For this review, take the finished solid that the model builds, in its own axes (mm). A direction names the side the tool comes from. Coordinates: 2 decimals unless noted, no trailing zeros. Loops run counter-clockwise (first coordinate to the right, second up) from the corner with the lowest first, then second, coordinate; pieces in that order, holes last. Notation, with made-up numbers: M 72.25,45.5 L 118.25,45.5 A17 ccw 118.25,68.5 Z; hole C -8,75 d9. An arc over 180 degrees is marked long. Answer as a JSON object with one key per item and string values. Group by question number.
Item 1: Add section B-B (y = 0). State the section outline as (x, z) points.
Item 2: Add section A-A (z = 6). State the section outline as (x, y) points.
Item 3: Tool access review of faces 1 (the face through (-13, -13, 20.7)), 2 (the face through (-17.8, 17.87, 10.49)): name each direction out of +Z, -Z, +X, -X, +Y, -Y from which nothing blocks a thin tool from reaching the whole face with its end or side.
Item 4: Mouldability with a two-part tool opening along Y and no side actions: class faces 3 (the face through (19.3, 0, 10)), 4 (the face through (17.264, -5.437, 26.468)), 5 (the face through (15.209, -13.523, 10.495)), 6 (the face through (-12.991, -13.523, 10.495)) as +Y half, -Y half, draft (parallel to the pull), parting line (faces both ways), or undercut.
Item 5: Wall thickness on L1, parallel to Y at x = 14.1, z = 5.5; L2, parallel to X at y = 15, z = 12.5: over which ranges is each line inside the solid? List them lowest first. Write a range as from..to.
Item 6: Insertion check: pin 1 (4 mm diameter, centred on x = -14.1, y = -14.1, fed in from +Z); pin 2 (2 mm diameter, centred on x = 14.1, y = -14.1, fed in from +Z); pin 3 (6 mm diameter, centred on x = 11, z = 30, fed in from +Y). Each pin has a flat end and moves straight along its axis. Give the tip position at first contact, or say it passes through.
Autodesk Inventor part; units mm, degrees
ref_plane "YZ Plane" through (0, 0, 0) normal (1, 0, 0) x (0, 1, 0)
ref_plane "XZ Plane" through (0, 0, 0) normal (0, 1, 0) x (-1, 0, 0)
ref_plane "XY Plane" through (0, 0, 0) normal (0, 0, 1) x (1, 0, 0)
sketch "スケッチ1" plane through (0, 0, 0) normal (0, 0, 1) x (1, 0, 0)
  line L0 (-19.3, -19.3) -> (19.3, -19.3)
  line L1 (19.3, -19.3) -> (19.3, 19.3)
  line L2 (19.3, 19.3) -> (-19.3, 19.3)
  line L3 (-19.3, 19.3) -> (-19.3, -19.3)
  line L4 (-19.3, -19.3) -> (19.3, 19.3) construction
  line L5 (19.3, -19.3) -> (-19.3, 19.3) construction
  point P0 (0, 0)
  dimension "d0" = 38.6
  dimension "d1" = 38.6
extrude "押し出し1" add sketch "スケッチ1" along normal blind 20.7
sketch "スケッチ2" plane through (0, 0, 20.7) normal (0, 0, 1) x (1, 0, 0)
  circle A0 centre (0, 0) radius 18.1
  dimension "d4" = 36.2
extrude "押し出し2" add sketch "スケッチ2" along normal blind 12.7
sketch "スケッチ3" plane through (0, 0, 0) normal (0, 0, -1) x (-1, 0, 0)
  line L0 (-14.1, -14.1) -> (14.1, -14.1) construction
  line L1 (14.1, -14.1) -> (14.1, 14.1) construction
  line L2 (14.1, 14.1) -> (-14.1, 14.1) construction
  line L3 (-14.1, 14.1) -> (-14.1, -14.1) construction
  line L4 (-14.1, -14.1) -> (14.1, 14.1) construction
  line L5 (14.1, -14.1) -> (-14.1, 14.1) construction
  point P0 (0, 0)
  dimension "d7" = 28.2
  dimension "d8" = 28.2
hole "穴1" at (-14.1, 14.1, 0) at (-14.1, -14.1, 0) at (14.1, -14.1, 0) at (14.1, 14.1, 0) direction (0, 0, 1) diameter 2.5 end through all
fillet "フィレット1" radius 5 4 edges at (19.3, 19.3, 10.35) (19.3, -19.3, 10.35) (-19.3, 19.3, 10.35) (-19.3, -19.3, 10.35)
chamfer "面取り1" distance 1 angle 45 1 edges at (-18.1, 0, 33.4)
properties part number "YDLiDAR_T-mini-pro"
From the geometry:
{
 "1": {"outline": "M -19.3,0 L 19.3,0 L 19.3,20.7 L 18.1,20.7 L 18.1,32.4 L 17.1,33.4 L -17.1,33.4 L -18.1,32.4 L -18.1,20.7 L -19.3,20.7 Z"},
 "2": {"outline": "M -19.3,-14.3 A5 ccw -14.3,-19.3 L 14.3,-19.3 A5 ccw 19.3,-14.3 L 19.3,14.3 A5 ccw 14.3,19.3 L -14.3,19.3 A5 ccw -19.3,14.3 Z; hole C -14.1,-14.1 d2.5; hole C -14.1,14.1 d2.5; hole C 14.1,-14.1 d2.5; hole C 14.1,14.1 d2.5"},
 "3": {"face 1": "+Z", "face 2": "+Z, -Z, -X, +Y"},
 "4": {"face 3": "draft", "face 4": "parting line", "face 5": "undercut", "face 6": "undercut"},
 "5": {"L1": "y = -19.3..-15.35, -12.85..12.85, 15.35..19.3", "L2": "x = -19.25..-14.97, -13.23..13.23, 14.97..19.25"},
 "6": {"pin 1": "stops at z = 32.56", "pin 2": "passes through", "pin 3": "stops at y = 16.24"}
}
